Drawing for the job (mm, zero at the part's lowest x, y, z). A direction names the side the tool comes from. Give positions to 0.01 mm unless a question says otherwise; leave off trailing zeros. Write each loop counter-clockwise with the first axis right and the second up, starting at its lowest first coordinate (ties: lowest second). Pieces come first, ordered by that corner, then holes. Notation, with made-up numbers: (57, -12) - (71, -12) arc R14 ccw to (71, 2) - close; hole circle Ø2 at (5.5, -11.75). An arc over 180 degrees is marked (long way). Use CSV: the item, a comma, the result in double quotes.
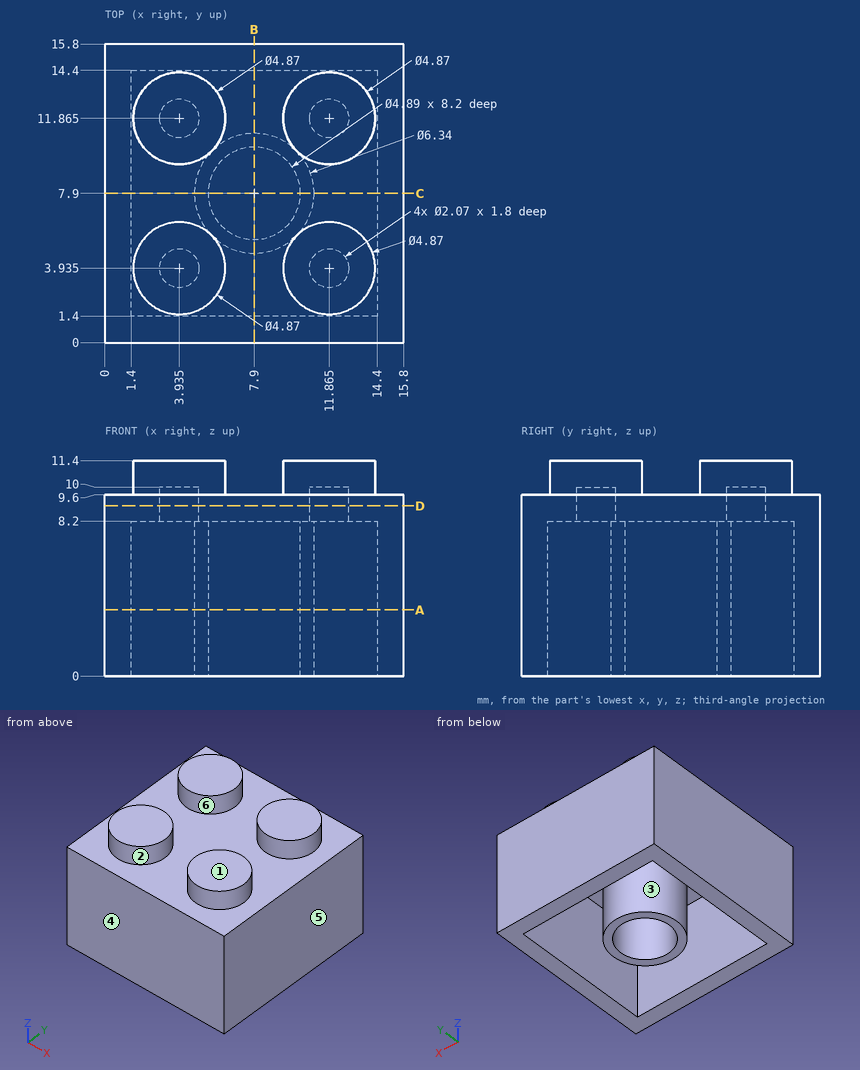
(1) Flat gauge pins, fed straight in: P1, Ø2, axis at x = 4, y = 7.5, coming from the +Z side; P2, Ø2.5, axis at x = 12.5, y = 12, coming from the -Z side. Where does each tip first touch, or does it go through?
Checked values:
P1,"stops at z = 9.6"
P2,"stops at z = 8.2"
(2) Saw through at B-B, the plane x = 7.9. List the corners of the cut face in (y, z) (3 decimals), then the cut area to 3 significant figures.
Checked values:
outline,"(0, 0) - (1.4, 0) - (1.4, 8.2) - (4.73, 8.2) - (4.73, 0) - (5.455, 0) - (5.455, 8.2) - (10.345, 8.2) - (10.345, 0) - (11.07, 0) - (11.07, 8.2) - (14.4, 8.2) - (14.4, 0) - (15.8, 0) - (15.8, 9.6) - (0, 9.6) - close"
area,"57.0 mm^2"
(3) 3-axis set-ups, long thin cutter, end or side, ignore diameter. For the marked faces 1, 2 and 3: which of +Z, -Z, +X, -X, +Y, -Y reach the whole face in a straight line?
Checked values:
face 1,"+Z, +X, -X, +Y, -Y"
face 2,"+Z"
face 3,"-Z"
(4) Pull direction Y, two halves, no side cores. Call the marked faces 4, 5 and 6: released by +Y, released by -Y, zero draft, split by the parting line, or undercut.
Checked values:
face 4,"released by -Y"
face 5,"zero draft"
face 6,"undercut"
(5) Wall check: probe 1 along Y at (x, z) = (7.9, 6.75) (3 decimals); probe 2 along Y at (x, z) = (2, 3); probe 3 along Y at (x, z) = (7.25, 7). Give the ranges that are in metal, low to high. Write a range as [from, to].
Checked values:
probe 1,"y = [0, 1.4], [4.73, 5.455], [10.345, 11.07], [14.4, 15.8]"
probe 2,"y = [0, 1.4], [14.4, 15.8]"
probe 3,"y = [0, 1.4], [4.8, 5.54], [10.26, 11], [14.4, 15.8]"
(6) Saw through at D-D, the plane z = 9. List the corners of the cut face in (x, y) (3 decimals).
Checked values:
outline,"(0, 0) - (15.8, 0) - (15.8, 15.8) - (0, 15.8) - close; hole circle Ø2.07 at (3.935, 3.935); hole circle Ø2.07 at (3.935, 11.865); hole circle Ø2.07 at (11.865, 3.935); hole circle Ø2.07 at (11.865, 11.865)"
(7) Saw through at A-A, the plane z = 3.5. List the corners of the cut face in (x, y) (3 decimals).
Checked values:
outline,"(0, 0) - (15.8, 0) - (15.8, 15.8) - (0, 15.8) - close; circle Ø6.34 at (7.9, 7.9); hole (1.4, 1.4) - (14.4, 1.4) - (14.4, 14.4) - (1.4, 14.4) - close; hole circle Ø4.89 at (7.9, 7.9)"
